from build123d import *

# Parameters (mm, degrees)
CROQUIS1_W                 = 7
CROQUIS1_H                 = 4.4
SALIENTE_EXTRUIR1_DEPTH    = 8
CROQUIS2_OUTSIDE_W         = 11.3
CROQUIS2_OUTSIDE_H         = 8.7
CROQUIS2_OUTSIDE_W_2       = 4
CROQUIS2_OUTSIDE_H_2       = 2.04309095
CORTAR_EXTRUIR1_DEPTH      = 4
REDONDEO1_R                = 1
CORTAR_EXTRUIR2_DEPTH      = 2.178454525
CORTAR_EXTRUIR2_DEPTH_BACK = 4.221545475


with BuildPart() as part:
    # Croquis1 → Saliente-Extruir1 (new body)
    with BuildSketch(Plane(origin=(0, 0, 0), x_dir=(1, 0, 0), z_dir=(0, 1, 0))):
        Rectangle(CROQUIS1_W, CROQUIS1_H)
    extrude(amount=SALIENTE_EXTRUIR1_DEPTH)

    # Croquis2 outside → Cortar-Extruir1 (cut)
    with BuildSketch(Plane(origin=(0, 8, 0), x_dir=(1, 0, 0), z_dir=(0, 1, 0))):
        Rectangle(CROQUIS2_OUTSIDE_W, CROQUIS2_OUTSIDE_H)
        Rectangle(CROQUIS2_OUTSIDE_W_2, CROQUIS2_OUTSIDE_H_2, mode=Mode.SUBTRACT)
    extrude(amount=-CORTAR_EXTRUIR1_DEPTH, mode=Mode.SUBTRACT)

    # Redondeo1
    redondeo1_edges = [part.edges().sort_by_distance(p)[0] for p in [
        (3.5, 2, 2.2),
        (-3.5, 2, 2.2),
        (-3.5, 2, -2.2),
        (3.5, 2, -2.2),
    ]]
    fillet(redondeo1_edges, radius=REDONDEO1_R)

    # Croquis3 → Cortar-Extruir2 (cut, two sides)
    with BuildSketch(Plane.XY.offset(1.021545475)) as cortar_extruir2_sk:
        Polygon((-30.213727446, 16.325583484), (-2, 8), (0, 7.409820379), (2, 8), (30.213727446, 16.325583484), (30.213727446, 75.158559162), (-30.213727446, 75.158559162), align=None)
    extrude(amount=CORTAR_EXTRUIR2_DEPTH, mode=Mode.SUBTRACT)
    extrude(cortar_extruir2_sk.sketch, amount=-CORTAR_EXTRUIR2_DEPTH_BACK, mode=Mode.SUBTRACT)


solid = part.part
The listing builds one solid part. Answer for the finished solid, in the listing's coordinates (mm). A direction names the side the tool comes from. Round coordinates to 2 decimals unless told otherwise and drop trailing zeros. Write each loop counter-clockwise with the first axis right and the second up, starting at its lowest first coordinate (ties: lowest second). Pieces come first, ordered by that corner, then holes. Notation, with made-up numbers: M 42,12.5 L 75,12.5 A27 cw 75,33.5 Z; hole C -4,7.25 d2. An arc over 180 degrees is marked long. Write each question's results on one line, items separated by ' | '. Start each with the question number.
Item 1: Straight lines are drawn through the part: probe 1 along Z at (x, y) = (-1.5, 5.75); probe 2 along Y at (x, z) = (2.75, 0.5); probe 3 along X at (y, z) = (7, 0.05). For each, find the intervals that lie inside material, in ascending order.
Item 2: Which of the six approach directions +Z, -Z, +X, -X, +Y, -Y give full straight-line access (tool end or side, diameter ignored) to faces 4 (the flat face through (0, 6, 1.022)), 5 (the flat face through (-2, 6, 0)), 6 (the flat face through (-1.014, 7.709, 0.014)), 7 (the flat face through (2, 6, 0))?
Item 3: Find section B-B on y = 2.75. Write down the section's boundary in (x, z).
Item 4: Find section D-D on z = -1.8. Write down the section's boundary in (x, y), and give its area (3 significant figures).
Item 5: Find section A-A on z = -0.4. Write down the section's boundary in (x, y), and give its area (3 significant figures).
Item 6: Given pin 1 Ø1 at (y, z) = (5.5, -0.5) entering from -X; pin 2 Ø2 at (x, y) = (0, 6.5) entering from +Z; pin 3 Ø1.2 at (x, y) = (0, 6.5) entering from -Z, each flat-ended and moving along its own axis, determine where each tip first touches the part or whether it passes through.
Item 7: Find section C-C on x = -1.25. Write down the section's boundary in (y, z).
Item 8: The mould has two halves that part along X. Classify faces 1 (the cylindrical face through (3.199, 2.028, 1.915)), 2 (the flat face through (0, 2, -2.2)), 3 (the flat face through (0.99, 7.7, 0.01)): +X half, -X half, draft (parallel to the pull), parting line (faces both ways), or undercut.
Answer block:
1) probe 1: z = -1.02 to 1.02 | probe 2: y = 0 to 4 | probe 3: x = -2 to 2
2) face 4: +Z, +X, -X, +Y | face 5: +Z, -Z, -X, +Y | face 6: +Z, -Z, +Y | face 7: +Z, -Z, +X, +Y
3) outline: M -3.5,-1.2 A1 ccw -2.5,-2.2 L 2.5,-2.2 A1 ccw 3.5,-1.2 L 3.5,1.2 A1 ccw 2.5,2.2 L -2.5,2.2 A1 ccw -3.5,1.2 Z
4) outline: M -3.3,0 L 3.3,0 L 3.3,4 L -3.3,4 Z | area: 26.4 mm²
5) outline: M -3.5,0 L 3.5,0 L 3.5,4 L 2,4 L 2,8 L 0,7.41 L -2,8 L -2,4 L -3.5,4 Z | area: 42.8 mm²
6) pin 1: stops at x = -2 | pin 2: stops at z = 1.02 | pin 3: stops at z = -1.02
7) outline: M 0,-2.2 L 4,-2.2 L 4,-1.02 L 7.78,-1.02 L 7.78,1.02 L 4,1.02 L 4,2.2 L 0,2.2 Z
8) face 1: +X half | face 2: draft | face 3: undercut
